Autodesk Fusion 360 part; units mm, degrees
sketch "Sketch1" plane through (0, 0, 0) normal (0, 0, 1) x (1, 0, 0)
  circle A0 centre (0, 0) radius 50.9
  line L0 (60, -60) -> (-60, -60)
  line L1 (-60, -60) -> (-60, 60)
  line L2 (-60, 60) -> (60, 60)
  line L3 (60, 60) -> (60, -60)
  line L4 (60, -60) -> (-60, 60) construction
  line L5 (-60, -60) -> (60, 60) construction
  dimension "d1" = 101.8
extrude "Extrude1" add sketch "Sketch1" along normal blind 4 contours A0 | L0 L1 L2 L3
sketch "Sketch2" plane through (0, 0, 4) normal (0, 0, 1) x (-1, 0, 0)
  line L0 (-60, -60) -> (60, -60)
  line L1 (60, -60) -> (60, 60)
  line L2 (60, 60) -> (-60, 60)
  line L3 (-60, 60) -> (-60, -60)
  circle A0 centre (0, 0) radius 50.9
  dimension "d4" = 101.8
extrude "Extrude2" cut sketch "Sketch2" against normal blind 1.8 contours A0
fillet "Fillet1" radius 15 4 edges at (60, -60, 2) (-60, -60, 2) (60, 60, 2) (-60, 60, 2)
Check sheet for the modelled part. Datum: model origin and axes. Units: mm. A direction names the side the tool comes from. Round coordinates to 2 decimals unless told otherwise and drop trailing zeros. Loops run counter-clockwise (first coordinate to the right, second up) from the corner with the lowest first, then second, coordinate; pieces in that order, holes last. Notation, with made-up numbers: (-7, 87) - (3, 87) arc R36 ccw to (3, 122) - close; hole circle Ø6 at (-13.75, 80). An arc over 180 degrees is marked (long way). Answer as a JSON object with one key per item and string values. Group by question number.
Q1. Sectioned sample at A-A, the plane z = 3.05. Enter the section's corners in (x, y), plus the area to 3 significant figures.
Q2. Mould release check, pull along X, two halves, no side actions. Record for faces 3 (the face through (-60, -1, 2)), 4 (the face through (-27.36, -42.92, 3.11)), 5 (the face through (1, -60, 2)): released by +X, released by -X, zero draft, split by the parting line, or undercut.
Q3. Gauge pin test, flat ends, axial feed: P1, Ø1, axis at x = 12, y = 24.5, coming from the -Z side; P2, Ø1.5, axis at x = -12, y = 37, coming from the +Z side. Record the tip position at first contact, or that the pin passes through.
Q4. Scan lines: line 1 along X through (y, z) = (0, 2.75); line 2 along Z through (x, y) = (30.5, -1.5). Record each from-to range of solid material in increasing order. Write a range as [from, to].
Q5. Sectioned sample at B-B, the plane y = 0. Enter the section's corners in (x, z).
Q6. Set-up check for faces 1 (the face through (60, 1, 2)), 2 (the face through (1, -1, 2.2)): record each of +Z, -Z, +X, -X, +Y, -Y from which the full face is reachable in a straight line by a thin tool's end or side.
Solution:
{
 "1": {"outline": "(-60, -45) arc R15 ccw to (-45, -60) - (45, -60) arc R15 ccw to (60, -45) - (60, 45) arc R15 ccw to (45, 60) - (-45, 60) arc R15 ccw to (-60, 45) - close; hole circle Ø101.8 at (0, 0)", "area": "6,070 mm²"},
 "2": {"face 3": "released by -X", "face 4": "undercut", "face 5": "zero draft"},
 "3": {"P1": "stops at z = 0", "P2": "stops at z = 2.2"},
 "4": {"line 1": "x = [-60, -50.9], [50.9, 60]", "line 2": "z = [0, 2.2]"},
 "5": {"outline": "(-60, 0) - (60, 0) - (60, 4) - (50.9, 4) - (50.9, 2.2) - (-50.9, 2.2) - (-50.9, 4) - (-60, 4) - close"},
 "6": {"face 1": "+Z, -Z, +X, +Y, -Y", "face 2": "+Z"}
}
